```python
from build123d import *

# Parameters (mm, degrees)
SKETCH1_W                   = 133.35
SKETCH1_H                   = 69.98
PLATFORM_THICKNESS_DEPTH    = 5
SKETCH2_R                   = 1.1
MOUNTING_HOLES_1_DEPTH      = 151.679868927
SKETCH4_R                   = 1.1
MOUNTING_HOLES_2_DEPTH      = 151.679868927
SKETCH3_W                   = 7.62
SKETCH3_H                   = 12.7
SKETCH3_H_2                 = 21.44
CABLE_MANAGEMENT_HOLE_DEPTH = 151.679868927


with BuildPart() as part:
    # Sketch1 → platform_thickness (new body)
    with BuildSketch(Plane(origin=(0, 0, 0), x_dir=(1, 0, 0), z_dir=(0, 1, 0))):
        with Locations((-66.675, 34.99)):
            Rectangle(SKETCH1_W, SKETCH1_H)
    extrude(amount=PLATFORM_THICKNESS_DEPTH)

    # Sketch2 → mounting_holes_1 (cut, through all)
    with BuildSketch(Plane(origin=(0, 5, 0), x_dir=(1, 0, 0), z_dir=(0, 1, 0))):
        with Locations(Location((-5.75, 38.88, 0), (0, 0, 270))):
            Circle(SKETCH2_R)
        with Locations(Location((-5.75, 5.86, 0), (0, 0, 270))):
            Circle(SKETCH2_R)
        with Locations(Location((-127.67, 5.86, 0), (0, 0, 270))):
            Circle(SKETCH2_R)
        with Locations(Location((-127.67, 64.29, 0), (0, 0, 270))):
            Circle(SKETCH2_R)
    extrude(amount=-MOUNTING_HOLES_1_DEPTH, mode=Mode.SUBTRACT)

    # Sketch4 → mounting_holes_2 (cut, through all)
    with BuildSketch(Plane(origin=(0, 5, 0), x_dir=(1, 0, 0), z_dir=(0, 1, 0))):
        with Locations(Location((-25.716666667, 49.04, 0), (0, 0, 270))):
            Circle(SKETCH4_R)
        with Locations(Location((-25.716666667, 20.94, 0), (0, 0, 270))):
            Circle(SKETCH4_R)
        with Locations(Location((-53.816666667, 49.04, 0), (0, 0, 270))):
            Circle(SKETCH4_R)
        with Locations(Location((-53.816666667, 20.94, 0), (0, 0, 270))):
            Circle(SKETCH4_R)
        with Locations(Location((-79.533333333, 49.04, 0), (0, 0, 270))):
            Circle(SKETCH4_R)
        with Locations(Location((-79.533333333, 20.94, 0), (0, 0, 270))):
            Circle(SKETCH4_R)
        with Locations(Location((-107.633333333, 49.04, 0), (0, 0, 270))):
            Circle(SKETCH4_R)
        with Locations(Location((-107.633333333, 20.94, 0), (0, 0, 270))):
            Circle(SKETCH4_R)
    extrude(amount=-MOUNTING_HOLES_2_DEPTH, mode=Mode.SUBTRACT)

    # Sketch3 → cable_management_hole (cut, through all)
    with BuildSketch(Plane(origin=(0, 5, 0), x_dir=(1, 0, 0), z_dir=(0, 1, 0))):
        with Locations((-8.03, 27.46)):
            Rectangle(SKETCH3_W, SKETCH3_H)
        with Locations((-8.03, 54.67)):
            Rectangle(SKETCH3_W, SKETCH3_H_2)
    extrude(amount=-CABLE_MANAGEMENT_HOLE_DEPTH, mode=Mode.SUBTRACT)


solid = part.part
```
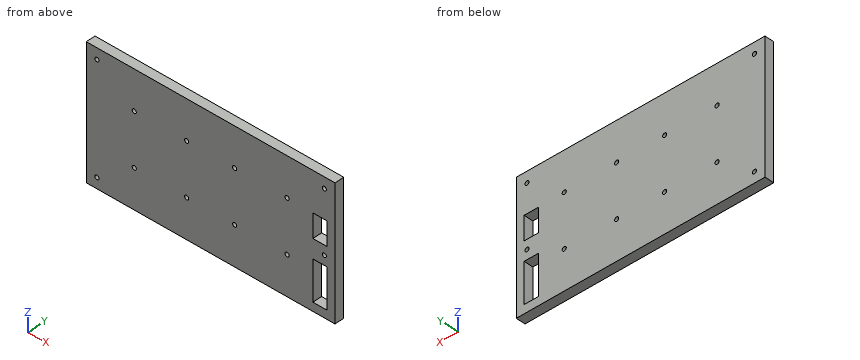
Verification items for the finished model (mm, model axes). Coordinates: 2 decimals unless noted, no trailing zeros. Loops run counter-clockwise (first coordinate to the right, second up) from the corner with the lowest first, then second, coordinate; pieces in that order, holes last. Notation, with made-up numbers: (-5, -14.75) - (39, -14.75) arc R33 cw to (39, 22.25) - close; hole circle Ø6 at (45.5, 46.5). An arc over 180 degrees is marked (long way). Return JSON: item names as keys, results as strings.
1. Section check A-A, the plane z = -23.5. Record the boundary of the cut face in (x, y), then the cut area to 3 significant figures.
Established:
{"outline": "(-133.35, 0) - (-11.84, 0) - (-11.84, 5) - (-133.35, 5) - close; (-4.22, 0) - (0, 0) - (0, 5) - (-4.22, 5) - close", "area": "629 mm2"}
2. Section check B-B, the plane y = 1.5. Count the separate pieces of the cut face and the enclosed holes in it, then the cut area to 3 significant figures.
Established:
{"separate pieces": "1", "enclosed holes": "14", "area": "9,030 mm2"}
3. Go/stop test with flat-tipped pins: pin 1 (1 mm diameter, centred on x = -46, z = -12.5, fed in from -Y); pin 2 (2 mm diameter, centred on x = -79.53, z = -49.04, fed in from +Y). Record where each tip stops, or that it passes through.
Established:
{"pin 1": "stops at y = 0", "pin 2": "passes through"}
4. Thickness scan on L1, parallel to Z at x = -9.5, y = 1.3; L2, parallel to X at y = 1, z = -5.86; L3, parallel to X at y = 2, z = -24. Record the ranges inside material, lowest first.
Established:
{"L1": "z = -69.98 to -65.39, -43.95 to -33.81, -21.11 to 0", "L2": "x = -133.35 to -128.77, -126.57 to -6.85, -4.65 to 0", "L3": "x = -133.35 to -11.84, -4.22 to 0"}
